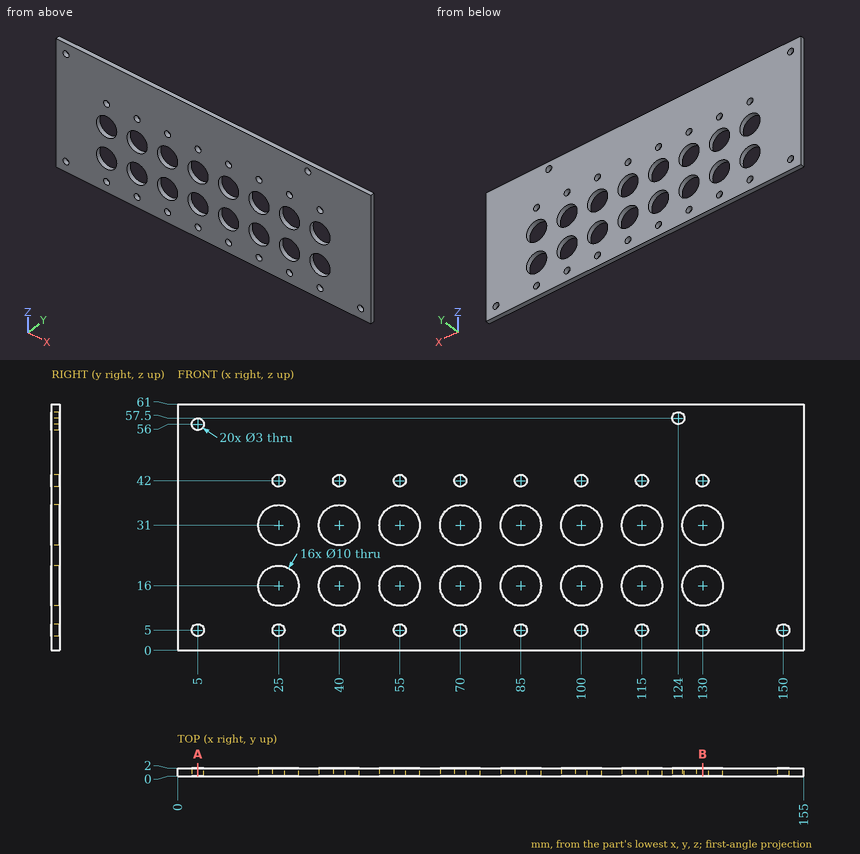
Drawing for the job (mm, zero at the part's lowest x, y, z). Round coordinates to 2 decimals unless told otherwise and drop trailing zeros. Write each loop counter-clockwise with the first axis right and the second up, starting at its lowest first coordinate (ties: lowest second). Pieces come first, ordered by that corner, then holes. Notation, with made-up numbers: M -6,72.5 L 37,72.5 A24 ccw 37,88.5 Z; hole C -2.75,63 d2. An arc over 180 degrees is marked long. Put each result on its own line as item: value.
Item 1: Cut at B-B (x = 130). List the corners of the cut face in (y, z), and give its area (3 significant figures).
Responses:
outline: M 0,0 L 2,0 L 2,3.5 L 0,3.5 Z; M 0,6.5 L 2,6.5 L 2,11 L 0,11 Z; M 0,21 L 2,21 L 2,26 L 0,26 Z; M 0,36 L 2,36 L 2,40.5 L 0,40.5 Z; M 0,43.5 L 2,43.5 L 2,61 L 0,61 Z
area: 70.0 mm²
Item 2: Cut at A-A (x = 5). List the corners of the cut face in (y, z).
Responses:
outline: M 0,0 L 2,0 L 2,3.5 L 0,3.5 Z; M 0,6.5 L 2,6.5 L 2,54.5 L 0,54.5 Z; M 0,57.5 L 2,57.5 L 2,61 L 0,61 Z
Item 3: Probe L1, parallel to Z at x = 25, y = 1.45; L2, parallel to Z at x = 104.5, y = 1.4. List the from-to ranges inside material, lowest first. Write a range as from..to.
Responses:
L1: 0..3.5, 6.5..11, 21..26, 36..40.5, 43.5..61
L2: 0..13.82, 18.18..28.82, 33.18..61
